Geometry: final body of the model. Coordinates: model frame, mm. Face numbers are marked on the shaded views. A direction names the side the tool comes from. Give positions to 0.01 mm unless a question says otherwise; leave off trailing zeros. Write each loop counter-clockwise with the first axis right and the second up, starting at its lowest first coordinate (ties: lowest second). Pieces come first, ordered by that corner, then holes.
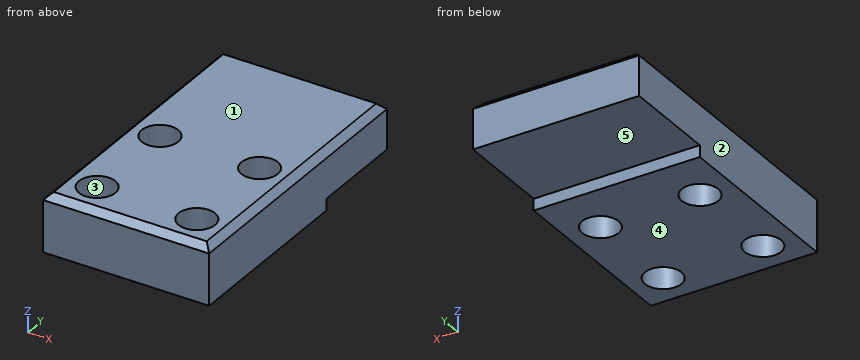
from build123d import *

# Parameters (mm, degrees)
SKETCH1_R           = 5.5
BOSS_EXTRUDE1_DEPTH = 3.5
SKETCH2_R           = 5.5
BOSS_EXTRUDE2_DEPTH = 14
CHAMFER1_SIZE       = 2


with BuildPart() as part:
    # Sketch1 → Boss-Extrude1 (new body)
    with BuildSketch(Plane.XY.offset(300)):
        Polygon((75, 66), (125, 66), (125, 60), (125, 50), (125, 10), (115, 10), (85, 10), (75, 10), (75, 50), (75, 60), align=None)
        with Locations((85, 50)):
            Circle(SKETCH1_R, mode=Mode.SUBTRACT)
        with Locations((115, 50)):
            Circle(SKETCH1_R, mode=Mode.SUBTRACT)
        with Locations((85, 20)):
            Circle(SKETCH1_R, mode=Mode.SUBTRACT)
        with Locations((115, 20)):
            Circle(SKETCH1_R, mode=Mode.SUBTRACT)
    extrude(amount=BOSS_EXTRUDE1_DEPTH)

    # Sketch2 → Boss-Extrude2 (add)
    with BuildSketch(Plane.XY.offset(303.5)):
        Polygon((75, 10), (75, 85), (75, 95), (125, 95), (125, 85), (125, 10), align=None)
        with Locations((85, 20)):
            Circle(SKETCH2_R, mode=Mode.SUBTRACT)
        with Locations((115, 20)):
            Circle(SKETCH2_R, mode=Mode.SUBTRACT)
        with Locations((115, 50)):
            Circle(SKETCH2_R, mode=Mode.SUBTRACT)
        with Locations((85, 50)):
            Circle(SKETCH2_R, mode=Mode.SUBTRACT)
    extrude(amount=BOSS_EXTRUDE2_DEPTH)

    # Chamfer1
    chamfer1_edges = [part.edges().sort_by_distance(p)[0] for p in [
        (100, 10, 317.5),
        (125, 52.5, 317.5),
        (100, 95, 317.5),
        (75, 52.5, 317.5),
    ]]
    chamfer(chamfer1_edges, length=CHAMFER1_SIZE)


solid = part.part
Q1. Section C-C on z = 310.5. Output: boundary loops of the cut face in (x, y).
Filled sheet:
outline: (75, 10) - (125, 10) - (125, 95) - (75, 95) - close; hole circle Ø11 at (85, 20); hole circle Ø11 at (85, 50); hole circle Ø11 at (115, 20); hole circle Ø11 at (115, 50)
Q2. Pin query (flat end, axial travel): P1, Ø8.5, axis at x = 88, y = 73.5, coming from the -Z side; P2, Ø10, axis at x = 115, y = 50, coming from the +Z side; P3, Ø3, axis at x = 108.5, z = 301.5, coming from the +Y side. Return the tip coordinate at first contact, or that it passes through.
Filled sheet:
P1: stops at z = 303.5
P2: passes through
P3: stops at y = 66
Q3. Access query for the marked faces 4 and 5. Directions: +Z, -Z, +X, -X, +Y, -Y. A direction counts if a zero-diameter tool reaches every point of the face in a straight line with its end or side. Return the directions, or none.
Filled sheet:
face 4: -Z, +X, -X, +Y, -Y
face 5: -Z, +X, -X, +Y
Q4. Ray query, line 1 along Y through (x, z) = (85, 311.5); line 2 along Y through (x, z) = (112.5, 303.25); line 3 along X through (y, z) = (48, 306.25). Return the intervals inside material, ascending.
Filled sheet:
line 1: y = 10 to 14.5, 25.5 to 44.5, 55.5 to 95
line 2: y = 10 to 15.1, 24.9 to 45.1, 54.9 to 66
line 3: x = 75 to 79.88, 90.12 to 109.88, 120.12 to 125
Q5. Section B-B on x = 85. Output: boundary loops of the cut face in (y, z).
Filled sheet:
outline: (10, 300) - (14.5, 300) - (14.5, 317.5) - (12, 317.5) - (10, 315.5) - close; (25.5, 300) - (44.5, 300) - (44.5, 317.5) - (25.5, 317.5) - close; (55.5, 300) - (66, 300) - (66, 303.5) - (95, 303.5) - (95, 315.5) - (93, 317.5) - (55.5, 317.5) - close
Q6. Pull-direction query (X, two-part tool) for the marked faces 1, 2 and 3; classes: released by +X, released by -X, zero draft, split by the parting line, or undercut.
Filled sheet:
face 1: zero draft
face 2: released by -X
face 3: undercut
Q7. Section A-A on y = 20. Output: boundary loops of the cut face in (x, z), plus the area to 3 significant figures.
Filled sheet:
outline: (75, 300) - (79.5, 300) - (79.5, 317.5) - (77, 317.5) - (75, 315.5) - close; (90.5, 300) - (109.5, 300) - (109.5, 317.5) - (90.5, 317.5) - close; (120.5, 300) - (125, 300) - (125, 315.5) - (123, 317.5) - (120.5, 317.5) - close
area: 486 mm2
Q8. Section D-D on y = 52. Output: boundary loops of the cut face in (x, z), plus the area to 3 significant figures.
Filled sheet:
outline: (75, 300) - (79.88, 300) - (79.88, 317.5) - (77, 317.5) - (75, 315.5) - close; (90.12, 300) - (109.88, 300) - (109.88, 317.5) - (90.12, 317.5) - close; (120.12, 300) - (125, 300) - (125, 315.5) - (123, 317.5) - (120.12, 317.5) - close
area: 512 mm2
